Drawing for the job (mm, zero at the part's lowest x, y, z). Coordinates: 2 decimals unless noted, no trailing zeros. Write each loop counter-clockwise with the first axis right and the second up, starting at its lowest first coordinate (ties: lowest second). Pieces come first, ordered by that corner, then holes. Notation, with made-up numbers: M 69.5,65.25 L 79.5,65.25 A15 cw 79.5,80.25 Z; hole C -34.75,27.25 d7. An arc over 180 degrees is marked long. Use CSV: the item, a comma, the result in double quotes. Start each with the question number.
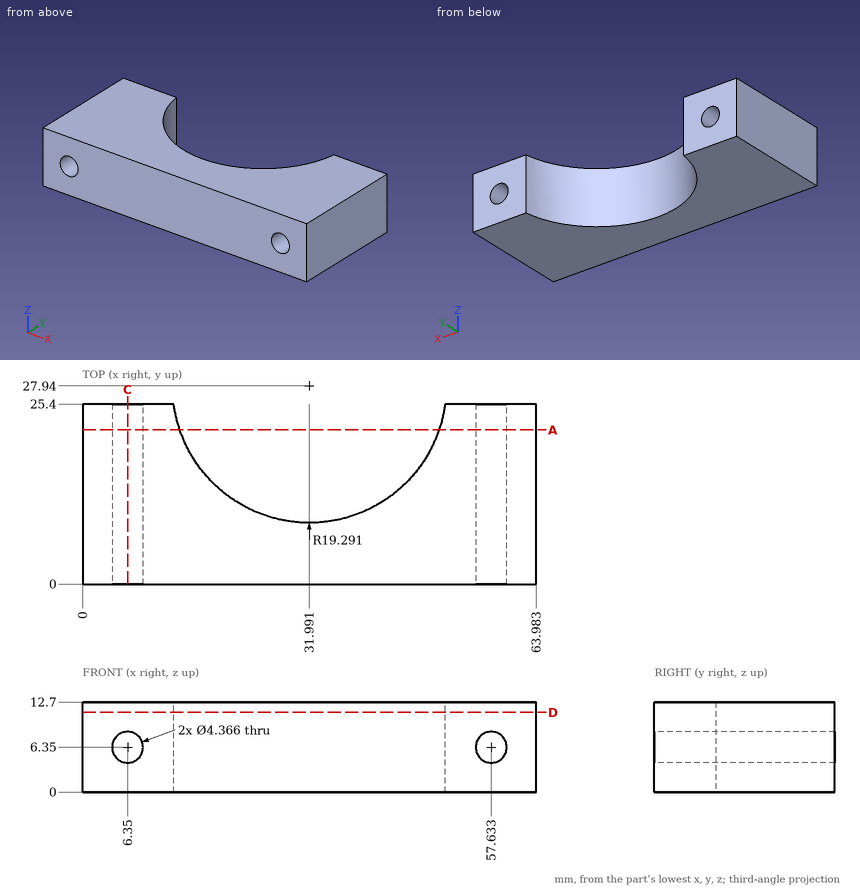
1) Drop flat-ended pins along their axis: P1, Ø1, axis at x = 22, z = 4, coming from the +Y side; P2, Ø3.5, axis at x = 57.63, z = 6.35, coming from the +Y side. Give the stop position or say it passes through.
2) Band-saw the part on D-D on z = 11.25. List the corners of the cut face in (x, y) (1 decimal).
3) Band-saw the part on C-C on x = 6.35. List the corners of the cut face in (y, z).
4) Wall check: L1, parallel to X at y = 19, z = 5 (1 decimal); L2, parallel to Z at x = 6.35, y = 9.25; L3, parallel to X at y = 17.5, z = 7.5 (1 decimal). Give the ranges that are in metal, low to high. Write a range as [from, to].
5) Band-saw the part on A-A on y = 21.75. State how many separate pieces and enclosed holes the cut face has.
Findings below:
1,P1,"stops at y = 11.75"
1,P2,"passes through"
2,outline,"M 0,0 L 64,0 L 64,25.4 L 51.1,25.4 A19.3 cw 12.9,25.4 L 0,25.4 Z"
3,outline,"M 0,0 L 25.4,0 L 25.4,4.17 L 0,4.17 Z; M 0,8.53 L 25.4,8.53 L 25.4,12.7 L 0,12.7 Z"
4,L1,"x = [0, 4.6], [8.1, 14.9], [49.1, 55.9], [59.3, 64]"
4,L2,"z = [0, 4.17], [8.53, 12.7]"
4,L3,"x = [0, 4.5], [8.2, 15.8], [48.2, 55.8], [59.5, 64]"
5,separate pieces,"2"
5,enclosed holes,"2"
